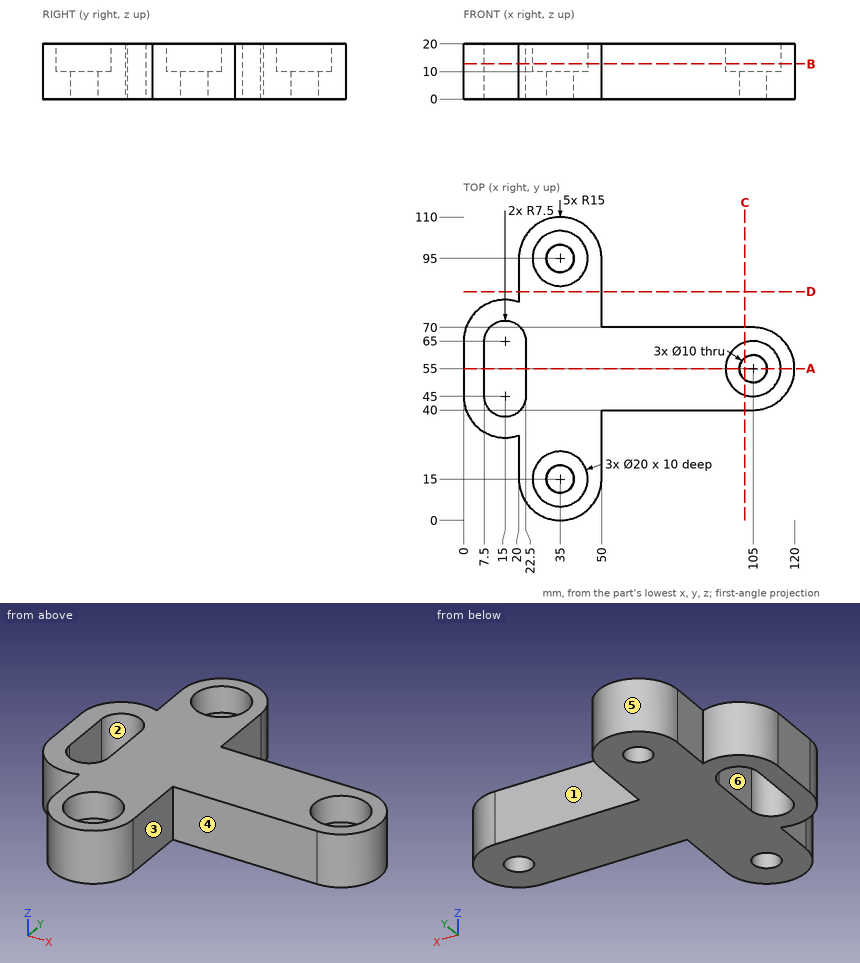
For this review, use the dimensioned drawing (mm, ordinates from the lowest corner) and the shaded views. A direction names the side the tool comes from. Round coordinates to 2 decimals unless told otherwise and drop trailing zeros. Loops run counter-clockwise (first coordinate to the right, second up) from the corner with the lowest first, then second, coordinate; pieces in that order, holes last. Notation, with made-up numbers: (50.25, -20.5) -> (87.25, -20.5) arc R22 cw to (87.25, 18.5) -> close; hole circle Ø3 at (-24.75, 79.25). An arc over 180 degrees is marked (long way). Write item = value, one per line. Start each with the question number.
Item 1: Insertion check: pin 1 (5 mm diameter, centred on y = 83.5, z = 13.5, fed in from -X); pin 2 (3 mm diameter, centred on x = 67, z = 16.5, fed in from -Y); pin 3 (6 mm diameter, centred on y = 31.5, z = 5.5, fed in from +X); pin 4 (22 mm diameter, centred on x = 108.5, y = 55, fed in from +Z). Each pin has a flat end and moves straight along its axis. Give the tip position at first contact, or say it passes through.
Item 2: To check wall thickness, follow L1, parallel to X at y = 15, z = 5.75; L2, parallel to Y at x = 105, z = 6; L3, parallel to Y at x = 105, z = 17.25. State the ranges of each line that lie inside material, in increasing order.
Item 3: Take a section at A-A on y = 55. Give the boundary of the cut face in (x, z), plus the area to 3 significant figures.
Item 4: Take a section at B-B on z = 12.75. Give the boundary of the cut face in (x, y).
Item 5: Take a section at C-C on x = 102. Give the boundary of the cut face in (y, z), plus the area to 3 significant figures.
Item 6: Mouldability with a two-part tool opening along Y and no side actions: class the marked faces 4, 5 and 6 as released by +Y, released by -Y, zero draft, split by the parting line, or undercut.
Item 7: Take a section at D-D on y = 83. Give the boundary of the cut face in (x, z), plus the area to 3 significant figures.
Item 8: For the marked faces 1, 2 and 3, list the 3-axis set-ups (+Z, -Z, +X, -X, +Y, -Y) from which the entire face can be reached by the end or side of a thin tool; tool diameter is ignored.
Result:
q1.pin_1 = 20
q1.pin_2 = 40
q1.pin_3 = 50
q1.pin_4 = 20
q2.L1 = 20 to 30, 40 to 50
q2.L2 = 40 to 50, 60 to 70
q2.L3 = 40 to 45, 65 to 70
q3.outline = (0, 0) -> (7.5, 0) -> (7.5, 20) -> (0, 20) -> close; (22.5, 0) -> (100, 0) -> (100, 10) -> (95, 10) -> (95, 20) -> (22.5, 20) -> close; (110, 0) -> (120, 0) -> (120, 20) -> (115, 20) -> (115, 10) -> (110, 10) -> close
q3.area = 1,800 mm²
q4.outline = (0, 45) arc R15 ccw to (20, 30.86) -> (20, 15) arc R15 ccw to (50, 15) -> (50, 40) -> (105, 40) arc R15 ccw to (105, 70) -> (50, 70) -> (50, 95) arc R15 ccw to (20, 95) -> (20, 79.14) arc R15 ccw to (0, 65) -> close; hole (7.5, 45) arc R7.5 ccw to (22.5, 45) -> (22.5, 65) arc R7.5 ccw to (7.5, 65) -> close; hole circle Ø20 at (35, 15); hole circle Ø20 at (35, 95); hole circle Ø20 at (105, 55)
q5.outline = (40, 0) -> (51, 0) -> (51, 10) -> (45.46, 10) -> (45.46, 20) -> (40, 20) -> close; (59, 0) -> (70, 0) -> (70, 20) -> (64.54, 20) -> (64.54, 10) -> (59, 10) -> close
q5.area = 329 mm²
q6.face_4 = released by -Y
q6.face_5 = released by +Y
q6.face_6 = undercut
q7.outline = (20, 0) -> (50, 0) -> (50, 20) -> (20, 20) -> close
q7.area = 600 mm²
q8.face_1 = +Z, -Z, +X, +Y
q8.face_2 = +Z, -Z
q8.face_3 = +Z, -Z, +X, -Y
